Can you work these out from the model? Positions are in its coordinate system, mm. Give positions to 0.01 mm unless a question says otherwise; leave off trailing zeros. Write each loop counter-clockwise with the first axis right and the second up, starting at its lowest first coordinate (ties: lowest second). Pieces come first, ordered by that corner, then holes. Notation, with made-up numbers: (58.5, 51.25) -> (63.5, 51.25) arc R22 ccw to (63.5, 88.25) -> close; hole circle Ø10 at (71, -40). An arc over 180 degrees is marked (long way). One line per item, written item: value.
from build123d import *

# Parameters (mm, degrees)
PAD_DEPTH       = 1
SKETCH_R        = 9
POCKET_DEPTH    = 1.001
POCKET001_DEPTH = 1.001


with BuildPart() as part:
    # Sketch007 → Pad (new body)
    with BuildSketch(Plane.XY):
        with BuildLine():
            Line((13.5, 15.5), (-13.5, 15.5))
            ThreePointArc((-15.469616, 17.152704), (-14.785575, 15.967911), (-13.5, 15.5))
            Line((-15.469616, 17.152704), (-16.153704, 21.03236))
            ThreePointArc((-16.153704, 21.03236), (-17.281843, 22.891476), (-19.369594, 23.5))
            Line((-19.369594, 23.5), (-26.098892, 22.911263))
            ThreePointArc((-26.098892, 22.911263), (-32.808142, 21.113525), (-38.497913, 17.129504))
            Line((-40.313708, 15.313708), (-38.497913, 17.129504))
            ThreePointArc((-40.313708, 15.313708), (-43.782073, 10.122935), (-45, 4))
            Line((-45, 4), (-45, 0))
            Line((-45, 0), (30.5, 0))
            Line((30.5, 0), (30.5, 10.677124))
            ThreePointArc((30.75, 11.338562), (30.564586, 11.030678), (30.5, 10.677124))
            ThreePointArc((30.75, 11.338562), (30.935414, 11.646447), (31, 12))
            Line((31, 17.015221), (31, 12))
            ThreePointArc((31, 17.015221), (29.702361, 19.964331), (26.651377, 21))
            Line((18.276649, 20.267306), (26.651377, 21))
            ThreePointArc((18.276649, 20.267306), (16.511345, 19.490554), (15.583693, 17.799667))
            Line((15.583693, 17.799667), (15.469616, 17.152704))
            ThreePointArc((13.5, 15.5), (14.785575, 15.967911), (15.469616, 17.152704))
        make_face()
        with BuildLine():
            Line((-20, 13), (-17, 13))
            ThreePointArc((-17, 13), (-16.25, 13.75), (-17, 14.5))
            Line((-20, 14.5), (-17, 14.5))
            ThreePointArc((-20, 14.5), (-20.75, 13.75), (-20, 13))
        make_face(mode=Mode.SUBTRACT)
        with BuildLine():
            Line((-1.5, 13), (1.5, 13))
            ThreePointArc((1.5, 13), (2.25, 13.75), (1.5, 14.5))
            Line((-1.5, 14.5), (1.5, 14.5))
            ThreePointArc((-1.5, 14.5), (-2.25, 13.75), (-1.5, 13))
        make_face(mode=Mode.SUBTRACT)
        with BuildLine():
            Line((17, 13), (20, 13))
            ThreePointArc((20, 13), (20.75, 13.75), (20, 14.5))
            Line((17, 14.5), (20, 14.5))
            ThreePointArc((17, 14.5), (16.25, 13.75), (17, 13))
        make_face(mode=Mode.SUBTRACT)
    pad = extrude(amount=PAD_DEPTH)

    # Mirrored: Pad across Sketch007 H_Axis
    add(pad.mirror(Plane.ZX))

    # Sketch (on Face5 of Mirrored) → Pocket (cut, through all)
    with BuildSketch(Plane.XY.offset(1)):
        Circle(SKETCH_R)
    extrude(amount=-POCKET_DEPTH, mode=Mode.SUBTRACT)

    # Sketch008 → Pocket001 (cut, through all)
    with BuildSketch(Plane.XY):
        with BuildLine():
            Line((-41.5, 2.732233), (-41.5, -2.732233))
            ThreePointArc((-41.5, -2.732233), (-39.956709, -5.041932), (-37.232233, -4.5))
            Line((-35.792893, -3.06066), (-37.232233, -4.5))
            ThreePointArc((-35.792893, -3.06066), (-35.57612, -2.736237), (-35.5, -2.353553))
            Line((-35.5, 2.353553), (-35.5, -2.353553))
            ThreePointArc((-35.5, 2.353553), (-35.57612, 2.736237), (-35.792893, 3.06066))
            Line((-37.232233, 4.5), (-35.792893, 3.06066))
            ThreePointArc((-37.232233, 4.5), (-39.956709, 5.041932), (-41.5, 2.732233))
        make_face()
    extrude(amount=POCKET001_DEPTH, mode=Mode.SUBTRACT)


solid = part.part
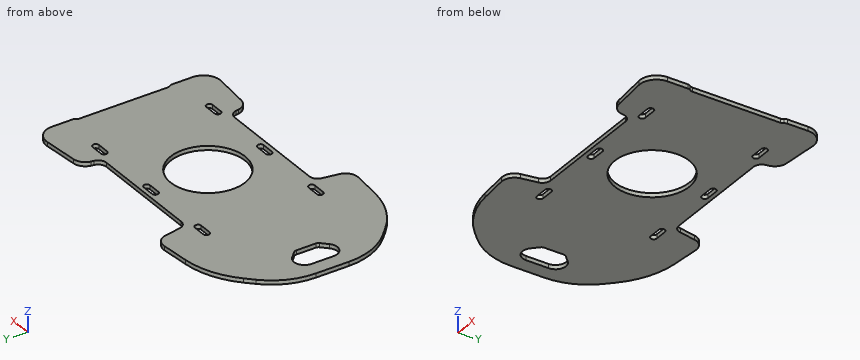
1) Will these pins go through, and if not, where does the flat tip stop? pin 1 (0.5 mm diameter, centred on x = -0.5, z = 0.5, fed in from +Y); pin 2 (12 mm diameter, centred on x = 2.5, y = 5, fed in from +Z); pin 3 (0.5 mm diameter, centred on y = 1, z = 0.5, fed in from +X); pin 4 (0.5 mm diameter, centred on x = -18, z = 0.5, fed in from +Y).
Answer list:
pin 1: stops at y = 15.5
pin 2: stops at z = 1
pin 3: stops at x = 30.5
pin 4: stops at y = 23.39
2) If we section it at B-B (x = 0): Write out the boundary of the cut face in (y, z).
Answer list:
outline: (-15.5, 0) -> (-14.5, 0) -> (-14.5, 1) -> (-15.5, 1) -> close; (-13, 0) -> (-9, 0) -> (-9, 1) -> (-13, 1) -> close; (9, 0) -> (13, 0) -> (13, 1) -> (9, 1) -> close; (14.5, 0) -> (15.5, 0) -> (15.5, 1) -> (14.5, 1) -> close
3) If we section it at C-C (y = 7): Write out the boundary of the cut face in (x, z).
Answer list:
outline: (-44.72, 0) -> (-5.66, 0) -> (-5.66, 1) -> (-44.72, 1) -> close; (5.66, 0) -> (30.5, 0) -> (30.5, 1) -> (5.66, 1) -> close
4) I need wall thicknesses on L1, parallel to Y at x = 0, z = 0.5; L2, parallel to X at y = 14, z = 0.1; L3, parallel to X at y = 5, z = 0.55. Which ranges of each line are inside material? Lowest first, please.
Answer list:
L1: y = -15.5 to -14.5, -13 to -9, 9 to 13, 14.5 to 15.5
L2: x = -41.49 to -20.71, -16.29 to -2.21, 2.21 to 16.29, 20.71 to 31
L3: x = -44.97 to -40.05, -37.95 to -7.48, 7.48 to 30.5
5) If we section it at D-D (x = -12): Write out the boundary of the cut face in (y, z), and give its area (3 significant figures).
Answer list:
outline: (-15.5, 0) -> (15.5, 0) -> (15.5, 1) -> (-15.5, 1) -> close
area: 31.0 mm^2
6) If we section it at A-A (y = 0): Write out the boundary of the cut face in (x, z).
Answer list:
outline: (-45, 0) -> (-41.5, 0) -> (-41.5, 1) -> (-45, 1) -> close; (-35.5, 0) -> (-9, 0) -> (-9, 1) -> (-35.5, 1) -> close; (9, 0) -> (30.5, 0) -> (30.5, 1) -> (9, 1) -> close
